The listing builds one solid part. Answer for the finished solid, in the listing's coordinates (mm). Face numbers are marked on the shaded views. A direction names the side the tool comes from. Give positions to 0.01 mm unless a question says otherwise; leave off trailing zeros. Loops run counter-clockwise (first coordinate to the right, second up) from the corner with the lowest first, then second, coordinate; pieces in that order, holes last.
Item 1: Section C-C, the plane y = 7.25 is taken. Give the vertices of the cut face in (x, z) (1 decimal), and give its area (3 significant figures).
Item 2: Each of these flat-tipped pins is pushed along its axis until it touches: pin 1 Ø4 at (x, y) = (1.5, -12.5) entering from -Z (3 decimals); pin 2 Ø3 at (y, z) = (-8.5, -0.5) entering from -X (3 decimals); pin 3 Ø3.5 at (x, z) = (0, 0) entering from -Y; pin 4 Ø2 at (y, z) = (1.5, 1.5) entering from +X. Where does it stop, or does it pass through?
Item 3: Consider line 1 along X through (y, z) = (-5.75, 0) (1 decimal); line 2 along Z through (x, y) = (2.75, -8); line 3 along Z through (x, y) = (-0.25, 6.25). Determine where each line is inside the solid, lowest interval first.
Item 4: The mould has two halves that part along X. Classify the marked faces 4, 5 and 6: pulls with the +X half, pulls with the -X half, needs draft (parallel to the pull), parting line crosses it, or undercut.
Item 5: A tool of negligible diameter and unlimited length cuts with its end or side. For the marked faces 1, 2 and 3, from which of +Z, -Z, +X, -X, +Y, -Y can it reach the whole face along a straight path? Write none if from no direction.
Item 6: Section A-A, the plane y = 3.5 is taken. Give the vertices of the cut face in (x, z) (1 decimal).
from build123d import *

# Parameters (mm, degrees)
BOSS_EXTRUDE1_DEPTH = 5.08
SKETCH2_R           = 2.54
BOSS_EXTRUDE2_DEPTH = 2.54
SKETCH4_R           = 2.921
SKETCH3_R           = 3.556
SKETCH7_R           = 3.175
BOSS_EXTRUDE3_DEPTH = 15.24
SKETCH8_R           = 1.5875
CUT_EXTRUDE1_DEPTH  = 26.316041239


with BuildPart() as part:
    # Sketch1 → Boss-Extrude1 (new body)
    with BuildSketch(Plane(origin=(0, 0, 0), x_dir=(1, 0, 0), z_dir=(0, 1, 0))):
        Polygon((2.199704526, 3.81), (-2.199704526, 3.81), (-4.399409051, 0), (-2.199704526, -3.81), (2.199704526, -3.81), (4.399409051, 0), align=None)
    extrude(amount=BOSS_EXTRUDE1_DEPTH)

    # Sketch2 → Boss-Extrude2 (add)
    with BuildSketch(Plane(origin=(0, 5.08, 0), x_dir=(1, 0, 0), z_dir=(0, 1, 0))):
        with Locations(Location((0, 0, 0), (0, 0, 270))):
            Circle(SKETCH2_R)
    extrude(amount=BOSS_EXTRUDE2_DEPTH)

    # Sketch4 → Loft1 section 0
    with BuildSketch(Plane(origin=(0, 9.398, 0), x_dir=(1, 0, 0), z_dir=(0, 1, 0))):
        Circle(SKETCH4_R)
    # Sketch3 → Loft1 section 1
    with BuildSketch(Plane(origin=(0, 7.62, 0), x_dir=(1, 0, 0), z_dir=(0, 1, 0))):
        Circle(SKETCH3_R)
    loft()

    # Sketch6 → Cut-Revolve1 (revolve, cut)
    with BuildSketch(Plane.XY):
        Polygon((4.399409051, 4.826), (3.764409051, 5.08), (4.399409051, 5.08), align=None)
        Polygon((4.399409051, 0), (4.399409051, 0.254), (3.764409051, 0), align=None)
    revolve(axis=Axis((0, 0, 0), (0, 1, 0)), mode=Mode.SUBTRACT)

    # Sketch7 → Boss-Extrude3 (add)
    with BuildSketch(Plane.XZ):
        with Locations(Location((0, 0, 0), (0, 0, 90))):
            Circle(SKETCH7_R)
    extrude(amount=BOSS_EXTRUDE3_DEPTH)

    # Sketch8 → Cut-Extrude1 (cut, through all)
    with BuildSketch(Plane(origin=(0, 9.398, 0), x_dir=(1, 0, 0), z_dir=(0, 1, 0))):
        with Locations(Location((0, 0, 0), (0, 0, 270))):
            Circle(SKETCH8_R)
    extrude(amount=-CUT_EXTRUDE1_DEPTH, mode=Mode.SUBTRACT)


solid = part.part
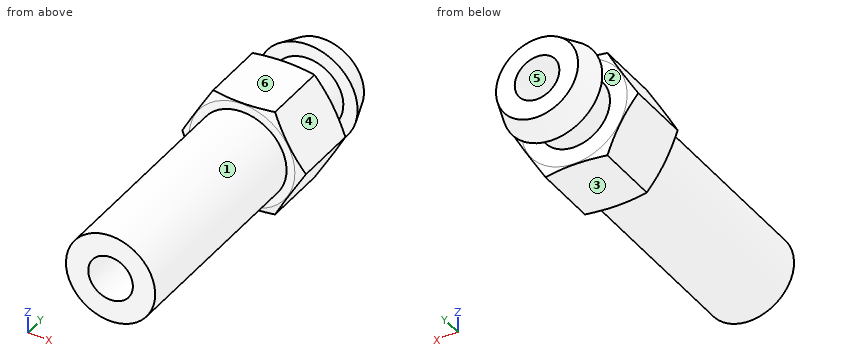
Worked answers:
1. outline: circle Ø5.1 at (0, 0); hole circle Ø3.2 at (0, 0)
1. area: 12.4 mm2
2. pin 1: stops at z = -3.175
2. pin 2: stops at x = -3.175
2. pin 3: stops at y = -15.24
2. pin 4: stops at x = 4.11
3. line 1: x = -3.2 to -1.6, 1.6 to 3.2
3. line 2: z = -1.59 to 1.59
3. line 3: z = -2.53 to -1.57, 1.57 to 2.53
4. face 4: pulls with the +X half
4. face 5: undercut
4. face 6: needs draft
5. face 1: -Y
5. face 2: none
5. face 3: -Z, +X, -X, +Y, -Y
6. outline: (-4.4, 0) - (-2.2, -3.8) - (2.2, -3.8) - (4.4, 0) - (2.2, 3.8) - (-2.2, 3.8) - close; hole circle Ø3.2 at (0, 0)
